from build123d import *

# Parameters (mm, degrees)
SKETCH1_R                = 2.4638
BOSS_EXTRUDE1_DEPTH      = 3.175
SKETCH5_R                = 3.175
SKETCH5_R_2              = 1.651
SKETCH5_R_3              = 1.4478
CUT_EXTRUDE2_DEPTH       = 4.175
SKETCH6_R                = 2.159
CUT_EXTRUDE3_DEPTH       = 4.175
SKETCH5_3_R              = 1.45415
CUT_EXTRUDE4_DEPTH       = 4.175
SKETCH5_4_R              = 1.5875
SKETCH5_4_R_2            = 4.7625
CUT_EXTRUDE5_DEPTH       = 4.175
SKETCH5_5_R              = 1.5875
CUT_EXTRUDE6_DEPTH       = 2.54
SKETCH5_6_R              = 1.5875
CUT_EXTRUDE7_DEPTH       = 4.175
SKETCH5_7_R              = 1.5875
SKETCH5_7_W              = 9.525
SKETCH5_7_H              = 19.05
CUT_EXTRUDE8_DEPTH       = 7.62
CUT_EXTRUDE8_DEPTH_BACK  = 2.54
SKETCH5_9_R              = 1.5875
CUT_EXTRUDE9_DEPTH       = 4.175
SKETCH5_15_R             = 2.159
SKETCH5_15_W             = 9.525
SKETCH5_15_H             = 19.05
CUT_EXTRUDE17_DEPTH      = 1
CUT_EXTRUDE17_DEPTH_BACK = 4.175
FILLET1_R                = 2.54
FILLET2_R                = 2.54
SKETCH2_R                = 1.9431
CUT_EXTRUDE20_DEPTH      = 4.175
FILLET3_R                = 2.54
FILLET4_R                = 2.54
SKETCH9_R                = 1.55
SKETCH9_R_2              = 2
CUT_EXTRUDE18_DEPTH      = 4.175
SKETCH3_R                = 1.5875
CUT_EXTRUDE19_DEPTH      = 976.122


with BuildPart() as part:
    # Sketch1 → Boss-Extrude1 (new body)
    with BuildSketch(Plane.XY):
        Polygon((-111.686526805, -95.25), (-127, -83.918625912), (-127, 83.918625912), (-111.686526805, 95.25), (111.686526805, 95.25), (127, 83.918625912), (127, -83.918625912), (111.686526805, -95.25), align=None)
        with Locations((-95.147512794, 56.885632681)):
            Circle(SKETCH1_R, mode=Mode.SUBTRACT)
        with Locations((-110.256011578, 77.303596941)):
            Circle(SKETCH1_R, mode=Mode.SUBTRACT)
        with Locations((110.256011578, 77.303596941)):
            Circle(SKETCH1_R, mode=Mode.SUBTRACT)
        with Locations((95.147512794, 56.885632681)):
            Circle(SKETCH1_R, mode=Mode.SUBTRACT)
        with Locations((-110.256011578, -77.303596941)):
            Circle(SKETCH1_R, mode=Mode.SUBTRACT)
        with Locations((-95.147512794, -56.885632681)):
            Circle(SKETCH1_R, mode=Mode.SUBTRACT)
        with Locations((110.256011578, -77.303596941)):
            Circle(SKETCH1_R, mode=Mode.SUBTRACT)
        with Locations((95.147512794, -56.885632681)):
            Circle(SKETCH1_R, mode=Mode.SUBTRACT)
    extrude(amount=BOSS_EXTRUDE1_DEPTH)

    # Sketch5 → Cut-Extrude2 (cut, through all)
    with BuildSketch(Plane(origin=(0, 0, 0), x_dir=(-1, 0, 0), z_dir=(0, 0, -1))):
        with BuildLine():
            Line((-25.4, -25.4), (-25.4, 25.4))
            ThreePointArc((-25.4, 25.4), (-28.575, 28.575), (-31.75, 25.4))
            Line((-31.75, 25.4), (-31.75, -25.4))
            ThreePointArc((-31.75, -25.4), (-28.575, -28.575), (-25.4, -25.4))
        make_face()
        with BuildLine():
            ThreePointArc((31.75, 25.4), (28.575, 28.575), (25.4, 25.4))
            Line((25.4, 25.4), (25.4, -25.4))
            ThreePointArc((25.4, -25.4), (28.575, -28.575), (31.75, -25.4))
            Line((31.75, -25.4), (31.75, 25.4))
        make_face()
        with Locations((82.55, 56.995822)):
            Circle(SKETCH5_R)
        with Locations((73.703688, 47.915322)):
            Circle(SKETCH5_R_2)
        with Locations((115.57, 47.915322)):
            Circle(SKETCH5_R_2)
        with Locations((73.703688, -47.915322)):
            Circle(SKETCH5_R_2)
        with Locations((115.57, -47.915322)):
            Circle(SKETCH5_R_2)
        with Locations((56.479426463, 15.03413)):
            Circle(SKETCH5_R_3)
        with Locations((56.479426463, -15.03413)):
            Circle(SKETCH5_R_3)
        with Locations((86.197426463, -15.03413)):
            Circle(SKETCH5_R_3)
        with Locations((86.197426463, 15.03413)):
            Circle(SKETCH5_R_3)
    extrude(amount=-CUT_EXTRUDE2_DEPTH, mode=Mode.SUBTRACT)

    # Sketch6 → Cut-Extrude3 (cut, through all)
    with BuildSketch(Plane(origin=(0, 0, 0), x_dir=(-1, 0, 0), z_dir=(0, 0, -1))):
        with Locations((-76.2, -85.725)):
            Circle(SKETCH6_R)
        with Locations((-25.4, -85.725)):
            Circle(SKETCH6_R)
        with Locations((25.4, -85.725)):
            Circle(SKETCH6_R)
        with Locations((76.2, -85.725)):
            Circle(SKETCH6_R)
        with Locations((76.2, 85.725)):
            Circle(SKETCH6_R)
        with Locations((25.4, 85.725)):
            Circle(SKETCH6_R)
        with Locations((-25.4, 85.725)):
            Circle(SKETCH6_R)
        with Locations((-76.2, 85.725)):
            Circle(SKETCH6_R)
        with Locations((117.475, -25.4)):
            Circle(SKETCH6_R)
        with Locations((117.475, 25.4)):
            Circle(SKETCH6_R)
        with Locations((-117.475, 25.4)):
            Circle(SKETCH6_R)
        with Locations((-117.475, -25.4)):
            Circle(SKETCH6_R)
    extrude(amount=-CUT_EXTRUDE3_DEPTH, mode=Mode.SUBTRACT)

    # Sketch5_3 → Cut-Extrude4 (cut, through all)
    with BuildSketch(Plane(origin=(0, 0, 0), x_dir=(-1, 0, 0), z_dir=(0, 0, -1))):
        with Locations((-42.5, 17.2)):
            Circle(SKETCH5_3_R)
        with Locations((-42.5, -17.2)):
            Circle(SKETCH5_3_R)
        with Locations((42.5, -17.2)):
            Circle(SKETCH5_3_R)
        with Locations((42.5, 17.2)):
            Circle(SKETCH5_3_R)
    extrude(amount=-CUT_EXTRUDE4_DEPTH, mode=Mode.SUBTRACT)

    # Sketch5_4 → Cut-Extrude5 (cut, through all)
    with BuildSketch(Plane(origin=(0, 0, 0), x_dir=(-1, 0, 0), z_dir=(0, 0, -1))):
        with Locations((61.544630637, -54.61)):
            Circle(SKETCH5_4_R)
        with Locations((61.544630637, -67.31)):
            Circle(SKETCH5_4_R)
        with Locations((-85.725, -85.725)):
            Circle(SKETCH5_4_R_2)
        with Locations((61.544630637, 54.61)):
            Circle(SKETCH5_4_R)
        with Locations((40.055369363, -67.31)):
            Circle(SKETCH5_4_R_2)
        with Locations((61.544630637, 67.31)):
            Circle(SKETCH5_4_R)
        with Locations((40.055369363, 67.31)):
            Circle(SKETCH5_4_R_2)
    extrude(amount=-CUT_EXTRUDE5_DEPTH, mode=Mode.SUBTRACT)

    # Sketch5_5 → Cut-Extrude6 (cut)
    with BuildSketch(Plane(origin=(0, 0, 0), x_dir=(-1, 0, 0), z_dir=(0, 0, -1))):
        with Locations((38.886108088, 54.61)):
            Circle(SKETCH5_5_R)
    extrude(amount=-CUT_EXTRUDE6_DEPTH, mode=Mode.SUBTRACT)

    # Sketch5_6 → Cut-Extrude7 (cut, through all)
    with BuildSketch(Plane(origin=(0, 0, 0), x_dir=(-1, 0, 0), z_dir=(0, 0, -1))):
        with Locations((38.886108088, 54.61)):
            Circle(SKETCH5_6_R)
    extrude(amount=-CUT_EXTRUDE7_DEPTH, mode=Mode.SUBTRACT)

    # Sketch5_7 → Cut-Extrude8 (cut, two sides)
    with BuildSketch(Plane(origin=(0, 0, 0), x_dir=(-1, 0, 0), z_dir=(0, 0, -1))) as cut_extrude8_sk:
        with Locations((40.055369363, -54.61)):
            Circle(SKETCH5_7_R)
        with Locations((-50.8, 76.2)):
            Rectangle(SKETCH5_7_W, SKETCH5_7_H)
    extrude(amount=CUT_EXTRUDE8_DEPTH, mode=Mode.SUBTRACT)
    extrude(cut_extrude8_sk.sketch, amount=-CUT_EXTRUDE8_DEPTH_BACK, mode=Mode.SUBTRACT)

    # Sketch5_9 → Cut-Extrude9 (cut, through all)
    with BuildSketch(Plane(origin=(0, 0, 0), x_dir=(-1, 0, 0), z_dir=(0, 0, -1))):
        with Locations((40.055369363, -54.61)):
            Circle(SKETCH5_9_R)
    extrude(amount=-CUT_EXTRUDE9_DEPTH, mode=Mode.SUBTRACT)

    # Sketch5_15 → Cut-Extrude17 (cut, two sides)
    with BuildSketch(Plane(origin=(0, 0, 0), x_dir=(-1, 0, 0), z_dir=(0, 0, -1))) as cut_extrude17_sk:
        with Locations((-74.93, -33.02)):
            Circle(SKETCH5_15_R)
        with Locations((-99.06, -33.02)):
            Circle(SKETCH5_15_R)
        with Locations((-99.06, 33.02)):
            Circle(SKETCH5_15_R)
        with Locations((-74.93, 33.02)):
            Circle(SKETCH5_15_R)
        with Locations((-50.8, 76.2)):
            Rectangle(SKETCH5_15_W, SKETCH5_15_H)
    extrude(amount=CUT_EXTRUDE17_DEPTH, mode=Mode.SUBTRACT)
    extrude(cut_extrude17_sk.sketch, amount=-CUT_EXTRUDE17_DEPTH_BACK, mode=Mode.SUBTRACT)

    # Fillet1
    fillet1_edges = [part.edges().sort_by_distance(p)[0] for p in [
        (55.5625, 85.725, 1.5875),
    ]]
    fillet(fillet1_edges, radius=FILLET1_R)

    # Fillet2
    fillet2_edges = [part.edges().sort_by_distance(p)[0] for p in [
        (46.0375, 85.725, 1.5875),
    ]]
    fillet(fillet2_edges, radius=FILLET2_R)

    # Sketch2 → Cut-Extrude20 (cut, through all)
    with BuildSketch(Plane.XY.offset(3.175)):
        with Locations((62.199353496, -76.2)):
            Circle(SKETCH2_R)
        with Locations((36.799353496, -76.2)):
            Circle(SKETCH2_R)
    extrude(amount=-CUT_EXTRUDE20_DEPTH, mode=Mode.SUBTRACT)

    # Fillet3
    fillet3_edges = [part.edges().sort_by_distance(p)[0] for p in [
        (46.0375, 66.675, 1.5875),
    ]]
    fillet(fillet3_edges, radius=FILLET3_R)

    # Fillet4
    fillet4_edges = [part.edges().sort_by_distance(p)[0] for p in [
        (55.5625, 66.675, 1.5875),
    ]]
    fillet(fillet4_edges, radius=FILLET4_R)

    # Sketch9 → Cut-Extrude18 (cut, through all)
    with BuildSketch(Plane.XY.offset(3.175)):
        with Locations((34.370000094, 30.350000006)):
            Circle(SKETCH9_R)
        with Locations((64.77, 30.350000006)):
            Circle(SKETCH9_R)
        with Locations((64.77, 6.35)):
            Circle(SKETCH9_R)
        with Locations((34.370000094, 6.35)):
            Circle(SKETCH9_R)
        with Locations((68.58, 69.85)):
            Circle(SKETCH9_R_2)
        with Locations((39.58, 69.85)):
            Circle(SKETCH9_R_2)
        with Locations((39.58, 42.35)):
            Circle(SKETCH9_R_2)
        with Locations((68.58, 42.35)):
            Circle(SKETCH9_R_2)
    extrude(amount=-CUT_EXTRUDE18_DEPTH, mode=Mode.SUBTRACT)

    # Sketch3 → Cut-Extrude19 (cut)
    with BuildSketch(Plane.XY.offset(3.175)):
        with Locations((-15.875, -65.560310834)):
            Circle(SKETCH3_R)
        with Locations((15.875, -65.560310834)):
            Circle(SKETCH3_R)
        with Locations((-15.875, -54.130310834)):
            Circle(SKETCH3_R)
        with Locations((15.875, -54.130310834)):
            Circle(SKETCH3_R)
    extrude(amount=-CUT_EXTRUDE19_DEPTH, mode=Mode.SUBTRACT)


solid = part.part
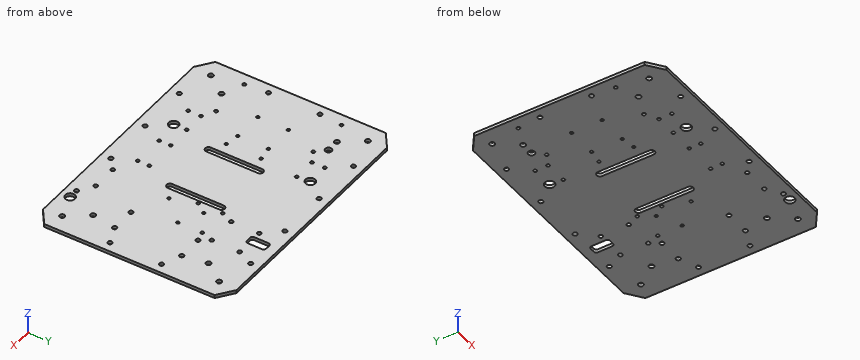
Here's how the part is built. I have some questions about the finished solid (model axes, mm). Coordinates: 2 decimals unless noted, no trailing zeros.
Item 1: If I drill on line 1 (X direction, y = -6.5, z = 1.8); line 2 (Y direction, x = -16, z = 0.9); line 3 (Y direction, x = 34.5, z = 0.7), over which ranges is the centre line in solid material (lowest first)?
Item 2: I want a section at A-A on z = 1.2. Count the separate pieces of the cut face and the enclosed holes in it, and give its area (3 significant figures).
Item 3: Will this pin go through, and if not, where does the flat tip stop? pin 1 (6.5 mm diameter, centred on x = 68.58, y = 42.35, fed in from -Z).
Findings below:
1. line 1: x = -127 to -31.75, -25.4 to 25.4, 31.75 to 127
1. line 2: y = -95.25 to -67.14, -63.98 to -55.71, -52.55 to 95.25
1. line 3: y = -95.25 to 4.81, 7.89 to 28.81, 31.89 to 95.25
2. separate pieces: 1
2. enclosed holes: 63
2. area: 46,300 mm2
3. pin 1: stops at z = 0
